```python
from build123d import *

# Parameters (mm, degrees)
SKETCH1_W           = 88.9
SKETCH1_H           = 28.284249084
BOSS_EXTRUDE1_DEPTH = 6.35
SKETCH2_W           = 6.35
SKETCH2_H           = 28.284249084
BOSS_EXTRUDE2_DEPTH = 25.4
SKETCH3_R           = 3.175
CUT_EXTRUDE1_DEPTH  = 6.35
SKETCH4_R           = 3.175
CUT_EXTRUDE2_DEPTH  = 7.62


with BuildPart() as part:
    # Sketch1 → Boss-Extrude1 (new body)
    with BuildSketch(Plane(origin=(0, 0, 0), x_dir=(1, 0, 0), z_dir=(0, 1, 0))):
        Rectangle(SKETCH1_W, SKETCH1_H)
    extrude(amount=BOSS_EXTRUDE1_DEPTH)

    # Sketch2 → Boss-Extrude2 (add)
    with BuildSketch(Plane(origin=(0, 6.35, 0), x_dir=(1, 0, 0), z_dir=(0, 1, 0))):
        with Locations((-41.275, 0)):
            Rectangle(SKETCH2_W, SKETCH2_H)
        with Locations((41.275, 0)):
            Rectangle(SKETCH2_W, SKETCH2_H)
    extrude(amount=BOSS_EXTRUDE2_DEPTH)

    # Sketch3 → Cut-Extrude1 (cut)
    with BuildSketch(Plane.ZY.offset(44.45)):
        with Locations((0, 19.247915812)):
            Circle(SKETCH3_R)
    extrude(amount=-CUT_EXTRUDE1_DEPTH, mode=Mode.SUBTRACT)

    # Sketch4 → Cut-Extrude2 (cut)
    with BuildSketch(Plane(origin=(44.45, 0, 0), x_dir=(0, 0, -1), z_dir=(1, 0, 0))):
        with Locations((0, 19.05)):
            Circle(SKETCH4_R)
    extrude(amount=-CUT_EXTRUDE2_DEPTH, mode=Mode.SUBTRACT)


solid = part.part
```
Geometry check sheet. Reference: the model listing, model coordinates, mm. A direction names the side the tool comes from. Coordinates: 2 decimals unless noted, no trailing zeros. Loops run counter-clockwise (first coordinate to the right, second up) from the corner with the lowest first, then second, coordinate; pieces in that order, holes last. Notation, with made-up numbers: (74.5, 11) - (117.5, 11) arc R13 cw to (117.5, 22) - close; hole circle Ø6 at (-33, 81). An arc over 180 degrees is marked (long way). One line per item, written item: value. Start each with the question number.
(1) Cross-section at A-A on y = 12. Enter the section's corners in (x, z), plus the area to 3 significant figures.
(2) Tool access check on faces 4 (the cylindrical face through (-41.32, 16.15, -0.69)), 5 (the flat face through (-44.45, 15.7, 0.2)), 6 (the flat face through (-1, 6.35, 0)). Record the directions out of +Z, -Z, +X, -X, +Y, -Y that give a thin tool (end or side, any length) a straight path to the whole face; none if there is none.
(3) Material ranges on line 1 (X direction, y = 17.5, z = 3.5); line 2 (Y direction, x = 42.5, z = 0) (3 decimals); line 3 (Y direction, x = -7.5, z = -0.5), recorded low to high. Write a range as [from, to].
(4) Cross-section at B-B on z = 0. Enter the section's corners in (x, y) (3 decimals).
(5) Depth check by flat-ended pin: P1, Ø3, axis at x = -31.5, z = 8, coming from the +Y side; P2, Ø5.5, axis at y = 19.05, z = 0, coming from the -X side; P3, Ø8.5, axis at y = 19.25, z = 0, coming from the +X side. Enter the tip coordinate at first touch or a pass-through.
(6) Cross-section at D-D on x = 25. Enter the section's corners in (y, z).
(7) Mould release check, pull along Z, two halves, no side actions. Record for faces 1 (the flat face through (-41, 31.75, 0)), 2 (the cylindrical face through (41.32, 15.95, 0.69)), 3 (the flat face through (-1, 5, -14.142)): released by +Z, released by -Z, zero draft, split by the parting line, or undercut.
(8) Cross-section at C-C on z = -10.5. Enter the section's corners in (x, y), plus the area to 3 significant figures.
Results below:
1. outline: (-44.45, -14.14) - (-38.1, -14.14) - (-38.1, 14.14) - (-44.45, 14.14) - close; (38.1, -14.14) - (44.45, -14.14) - (44.45, 14.14) - (38.1, 14.14) - close
1. area: 359 mm2
2. face 4: -X
2. face 5: +Z, -Z, -X, +Y, -Y
2. face 6: +Z, -Z, +Y
3. line 1: x = [-44.45, -38.1], [38.1, 44.45]
3. line 2: y = [0, 15.875], [22.225, 31.75]
3. line 3: y = [0, 6.35]
4. outline: (-44.45, 0) - (44.45, 0) - (44.45, 15.875) - (38.1, 15.875) - (38.1, 6.35) - (-38.1, 6.35) - (-38.1, 16.073) - (-44.45, 16.073) - close; (-44.45, 22.423) - (-38.1, 22.423) - (-38.1, 31.75) - (-44.45, 31.75) - close; (38.1, 22.225) - (44.45, 22.225) - (44.45, 31.75) - (38.1, 31.75) - close
5. P1: stops at y = 6.35
5. P2: passes through
5. P3: stops at x = 44.45
6. outline: (0, -14.14) - (6.35, -14.14) - (6.35, 14.14) - (0, 14.14) - close
7. face 1: zero draft
7. face 2: undercut
7. face 3: released by -Z
8. outline: (-44.45, 0) - (44.45, 0) - (44.45, 31.75) - (38.1, 31.75) - (38.1, 6.35) - (-38.1, 6.35) - (-38.1, 31.75) - (-44.45, 31.75) - close
8. area: 887 mm2
